Part model, mm, in its own coordinate system. A direction names the side the tool comes from. Round coordinates to 2 decimals unless told otherwise and drop trailing zeros. Loops run counter-clockwise (first coordinate to the right, second up) from the corner with the lowest first, then second, coordinate; pieces in that order, holes last. Notation, with made-up numbers: M 79.25,14 L 117.25,14 A27 cw 117.25,30 Z; hole C 81.5,19.5 d9. An arc over 180 degrees is marked long. Answer as CSV lines item,"result". Start each with the question number.
Item 1: Drop flat-ended pins along their axis: pin 1 Ø1 at (x, z) = (1.5, 8) entering from -Y; pin 2 Ø0.6 at (x, z) = (-0.5, 8) entering from -Y. Give the stop position or say it passes through.
Item 2: Band-saw the part on C-C (y = -4.5). Give the cut face in (x, z).
Item 3: Band-saw the part on D-D (x = -0.55). Give the cut face in (y, z).
Item 4: Band-saw the part on B-B (z = 5.75). Give the cut face in (x, y), and give its area (3 significant figures).
Item 5: Mould opens along Z. For faces 1 (the flat face through (-1.41, 1, 7)), 2 (the flat face through (-1, -3.16, 7)), 3 (the flat face through (-2.85, 0, 6)), 4 (the flat face through (0, 0, 13.11)) say: pulls with the +Z half, pulls with the -Z half, needs draft (parallel to the pull), parting line crosses it, or undercut.
Item 6: Wall check: line 1 (Z direction, x = -0.6, y = 4.5); line 2 (X direction, y = 1.5, z = 11.25); line 3 (Z direction, x = 0.5, y = 1.75). Give the ranges that are in metal, low to high.
Item 7: Which spindle directions (+Z, -Z, +X, -X, +Y, -Y) get a long thin tool onto all of the face, cutting with end or side? Do faces 5 (the flat face through (2.85, 0, 6)), 6 (the flat face through (-2.54, 0, 6)). Say none if no direction does.
Item 8: Band-saw the part on A-A (y = -3). Give the cut face in (x, z), and give its area (3 significant figures).
Autodesk Inventor part; units mm, degrees
ref_plane "YZ Plane" through (0, 0, 0) normal (1, 0, 0) x (0, 1, 0)
ref_plane "XZ Plane" through (0, 0, 0) normal (0, 1, 0) x (-1, 0, 0)
ref_plane "XY Plane" through (0, 0, 0) normal (0, 0, 1) x (1, 0, 0)
sketch "Skizze1" plane through (0, 0, 0) normal (0, 0, 1) x (1, 0, 0)
  line L0 (-2.85, 5.47) -> (2.85, 5.47)
  line L1 (2.85, 5.47) -> (2.85, -5.47)
  line L2 (2.85, -5.47) -> (-2.85, -5.47)
  line L3 (-2.85, -5.47) -> (-2.85, 5.47)
  line L4 (-2.85, 5.47) -> (2.85, -5.47) construction
  point P0 (0, 0)
  point P1 (0, 0)
  dimension "d0" = 5.7
  dimension "d1" = 10.94
extrude "Extrusion1" add sketch "Skizze1" along normal blind 13.11
shell "Wandung1" thickness 0.31 removed faces 1 at (0.95, -5.47, 4.37)
fillet "Rundung1" radius 0.1 8 edges at (2.85, 0, 13.11) (-2.85, 0, 13.11) (2.85, 0, 0) (-2.85, 0, 0) (2.54, -0.155, 12.8) (-2.54, -0.155, 12.8) (-2.54, -0.155, 0.31) (2.54, -0.155, 0.31)
sketch "Skizze2" plane through (-2.44, 5.16, 12.8) normal (0, -1, 0) x (1, 0, 0)
  arc A0 (4.88, -12.49) -> (4.98, -12.39) centre (4.88, -12.39) ccw construction
  line L0 (4.88, -12.39) -> (2.3, -12.39) construction
  line L1 (2.3, -12.39) -> (2.3, -11.55) construction
  line L2 (2.3, -11.55) -> (4.88, -11.55) construction
  line L3 (4.88, -11.55) -> (4.88, -12.39) construction
  arc A1 (4.98, -0.1) -> (4.88, 0) centre (4.88, -0.1) ccw construction
  line L4 (4.88, -0.1) -> (2.3, -0.1) construction
  line L5 (2.3, -0.1) -> (2.3, -0.94) construction
  line L6 (2.3, -0.94) -> (4.88, -0.94) construction
  line L7 (4.88, -0.94) -> (4.88, -0.1) construction
  line L8 (-0.1, -12.39) -> (-0.1, -0.1) construction
  line L9 (-0.1, -6.245) -> (1.03, -6.245) construction
  line L10 (2.3, -0.94) -> (1.03, -0.94)
  line L11 (1.03, -0.94) -> (1.03, -11.55)
  line L12 (1.03, -11.55) -> (2.3, -11.55)
  line L13 (2.3, -11.55) -> (2.3, -0.94)
  point P0 (2.44, -12.8)
  dimension "d6" = 2.58
  dimension "d7" = 0.84
  dimension "d8" = 2.58
  dimension "d9" = 0.84
  dimension "d10" = 1.13
extrude "Extrusion2" add sketch "Skizze2" along normal blind 8.32
properties part number "USBstick_halter"
Answer block:
1,pin 1,"stops at y = 5.16"
1,pin 2,"stops at y = -3.16"
2,outline,"M -2.85,0.1 A0.1 ccw -2.75,0 L 2.75,0 A0.1 ccw 2.85,0.1 L 2.85,13.01 A0.1 ccw 2.75,13.11 L -2.75,13.11 A0.1 ccw -2.85,13.01 Z; hole M -2.54,0.41 A0.1 ccw -2.44,0.31 L 2.44,0.31 A0.1 ccw 2.54,0.41 L 2.54,12.7 A0.1 ccw 2.44,12.8 L -2.44,12.8 A0.1 ccw -2.54,12.7 Z"
3,outline,"M -5.47,0 L 5.47,0 L 5.47,13.11 L -5.47,13.11 L -5.47,12.8 L 5.16,12.8 L 5.16,11.86 L -3.16,11.86 L -3.16,1.25 L 5.16,1.25 L 5.16,0.31 L -5.47,0.31 Z"
4,outline,"M -2.85,-5.47 L -2.54,-5.47 L -2.54,5.16 L -1.41,5.16 L -1.41,-3.16 L -0.14,-3.16 L -0.14,5.16 L 2.54,5.16 L 2.54,-5.47 L 2.85,-5.47 L 2.85,5.47 L -2.85,5.47 Z"
4,area,"18.9 mm^2"
5,face 1,"undercut"
5,face 2,"undercut"
5,face 3,"needs draft"
5,face 4,"pulls with the +Z half"
6,line 1,"z = 0 to 0.31, 1.25 to 11.86, 12.8 to 13.11"
6,line 2,"x = -2.85 to -2.54, -1.41 to -0.14, 2.54 to 2.85"
6,line 3,"z = 0 to 0.31, 12.8 to 13.11"
7,face 5,"+Z, -Z, +X, +Y, -Y"
7,face 6,"-Y"
8,outline,"M -2.85,0.1 A0.1 ccw -2.75,0 L 2.75,0 A0.1 ccw 2.85,0.1 L 2.85,13.01 A0.1 ccw 2.75,13.11 L -2.75,13.11 A0.1 ccw -2.85,13.01 Z; M -1.41,1.25 L -0.14,1.25 L -0.14,11.86 L -1.41,11.86 Z; hole M -2.54,0.41 A0.1 ccw -2.44,0.31 L 2.44,0.31 A0.1 ccw 2.54,0.41 L 2.54,12.7 A0.1 ccw 2.44,12.8 L -2.44,12.8 A0.1 ccw -2.54,12.7 Z"
8,area,"24.8 mm^2"
